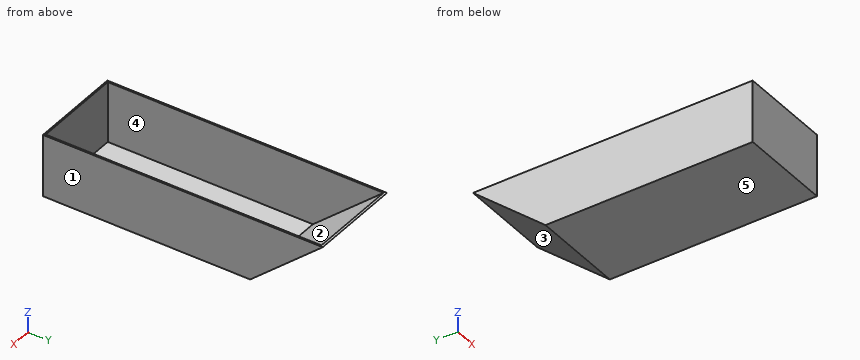
```python
from build123d import *

# Parameters (mm, degrees)
F1_DEPTH = 180
F2_T     = -3


with BuildPart() as f1:
    # F0 (on Right) → F1 (new body)
    with BuildSketch(Plane.YZ):
        Polygon((-200, 60), (-200, -60), (200, -60), (340, 60), (200, 60), align=None)
    extrude(amount=F1_DEPTH)

    # F2
    f2_openings = [f1.faces().sort_by_distance(p)[0] for p in [
        (90, 70, 60),
    ]]
    offset(amount=F2_T, openings=f2_openings)


solid = f1.part
```
Geometry: final body of the model. Coordinates: model frame, mm. Face numbers are marked on the shaded views. A direction names the side the tool comes from. Round coordinates to 2 decimals unless told otherwise and drop trailing zeros. Loops run counter-clockwise (first coordinate to the right, second up) from the corner with the lowest first, then second, coordinate; pieces in that order, holes last. Notation, with made-up numbers: (75.25, -20) -> (123.25, -20) arc R21 cw to (123.25, -14) -> close; hole circle Ø7 at (-19.5, 2.25). An arc over 180 degrees is marked (long way). Use one line per item in the form item = value. Start each with the question number.
1) Line query: L1, parallel to X at y = 166, z = -44; L2, parallel to Z at x = 66, y = -58.5; L3, parallel to Y at x = 153.5, z = -12. Output: solid intervals per line, ascending.
2) Section C-C on x = 23.5. Output: boundary loops of the cut face in (y, z).
3) Section D-D on z = -2. Output: boundary loops of the cut face in (x, y).
4) Draft query along Y for the marked faces 3, 4 and 5. Return one class per face: released by +Y, released by -Y, zero draft, split by the parting line, or undercut.
5) Section B-B on y = -2.5. Output: boundary loops of the cut face in (x, z), then the cut area to 3 significant figures.
6) Section A-A on z = 25. Output: boundary loops of the cut face in (x, y), then the cut area to 3 significant figures.
7) First-contact query: P1, Ø5, axis at x = 107.5, y = -94.5, coming from the +Z side; P2, Ø2, axis at x = 48.5, z = -46.5, coming from the +Y side; P3, Ø4, axis at x = 38, y = 241, coming from the -Z side. Flat tips, straight axial feed; report the tip coordinate or a pass-through.
8) Access query for the marked faces 1 and 2. Directions: +Z, -Z, +X, -X, +Y, -Y. A direction counts if a zero-diameter tool reaches every point of the face in a straight line with its end or side. Return the directions, or none.
Response:
q1.L1 = 0 to 3, 177 to 180
q1.L2 = -60 to -57
q1.L3 = -200 to -197, 251.39 to 256
q2.outline = (-200, -60) -> (200, -60) -> (340, 60) -> (335.39, 60) -> (198.89, -57) -> (-197, -57) -> (-197, 60) -> (-200, 60) -> close
q3.outline = (0, -200) -> (180, -200) -> (180, 267.67) -> (0, 267.67) -> close; hole (3, -197) -> (177, -197) -> (177, 263.06) -> (3, 263.06) -> close
q4.face_3 = released by +Y
q4.face_4 = undercut
q4.face_5 = zero draft
q5.outline = (0, -60) -> (180, -60) -> (180, 60) -> (177, 60) -> (177, -57) -> (3, -57) -> (3, 60) -> (0, 60) -> close
q5.area = 1,240 mm^2
q6.outline = (0, -200) -> (180, -200) -> (180, 299.17) -> (0, 299.17) -> close; hole (3, -197) -> (177, -197) -> (177, 294.56) -> (3, 294.56) -> close
q6.area = 4,320 mm^2
q7.P1 = -57
q7.P2 = 216.92
q7.P3 = -26.57
q8.face_1 = +Z, -Z, +X, +Y, -Y
q8.face_2 = +Z
